For this review, take the finished solid that the model builds, in its own axes (mm). A direction names the side the tool comes from. Give positions to 0.01 mm unless a question says otherwise; leave off trailing zeros. Write each loop counter-clockwise with the first axis right and the second up, starting at its lowest first coordinate (ties: lowest second). Pieces come first, ordered by that corner, then holes. Notation, with made-up numbers: M 40.5,-22 L 64.5,-22 A28 ccw 64.5,-4 Z; hole C 9.25,-25.75 d2. An arc over 180 degrees is marked long. One line per item, written item: value. Start each with the question number.
Item 1: Clearance check with flat-ended pins moving along their axes: pin 1 Ø2 at (y, z) = (0.5, -5) entering from -X; pin 2 Ø8 at (x, z) = (6, 2) entering from +Y; pin 3 Ø2 at (x, y) = (5, 1.5) entering from +Z; pin 4 Ø2 at (x, y) = (2, 0.5) entering from +Z. State where each tip first meets the part, or that it passes through.
Item 2: Consider section B-B, the plane x = 0. Write out the cut boundary in (y, z), and give its area (3 significant figures).
Item 3: Consider section A-A, the plane z = 0. Write out the cut boundary in (x, y), and give its area (3 significant figures).
Item 4: To check wall thickness, follow probe 1 along Z at (x, y) = (0, 3.45); probe 2 along Z at (x, y) = (0, 1.2). State the ranges of each line that lie inside material, in increasing order.
Item 5: Tool access review of faces 4 (the face through (6, 3.4, -2)), 5 (the face through (6, 0.1, -2)), 6 (the face through (7, 3.5, -2)): name each direction out of +Z, -Z, +X, -X, +Y, -Y from which nothing blocks a thin tool from reaching the whole face with its end or side.
Item 6: Mouldability with a two-part tool opening along X and no side actions: class faces 1 (the face through (-4, 0, -4)), 2 (the face through (-7.493, 1.726, -0.33)), 3 (the face through (-1.08, 1.73, 4.88)) as released by +X, released by -X, zero draft, split by the parting line, or undercut.
Item 7: Consider section C-C, the plane y = 2. Write out the cut boundary in (x, z), and give its area (3 significant figures).
Item 8: Consider section D-D, the plane z = 6.75. Write out the cut boundary in (x, y), and give its area (3 significant figures).
```python
from build123d import *

# Parameters (mm, degrees)
SKETCH1_R           = 7.5
SKETCH1_R_2         = 7
BOSS_EXTRUDE1_DEPTH = 3.5
SKETCH6_R           = 7
SKETCH6_R_2         = 6
BOSS_EXTRUDE4_DEPTH = 3.3
SKETCH7_R           = 6
SKETCH7_R_2         = 5
BOSS_EXTRUDE5_DEPTH = 3.5


with BuildPart() as part:
    # Sketch1 → Boss-Extrude1 (new body)
    with BuildSketch(Plane(origin=(0, 0, 0), x_dir=(1, 0, 0), z_dir=(0, 1, 0))):
        Circle(SKETCH1_R)
        Circle(SKETCH1_R_2, mode=Mode.SUBTRACT)
    extrude(amount=BOSS_EXTRUDE1_DEPTH)

    # Sketch6 → Boss-Extrude4 (add)
    with BuildSketch(Plane(origin=(0, 0.1, 0), x_dir=(1, 0, 0), z_dir=(0, 1, 0))):
        Circle(SKETCH6_R)
        Circle(SKETCH6_R_2, mode=Mode.SUBTRACT)
    extrude(amount=BOSS_EXTRUDE4_DEPTH)

    # Sketch7 → Boss-Extrude5 (add)
    with BuildSketch(Plane(origin=(0, 0, 0), x_dir=(1, 0, 0), z_dir=(0, 1, 0))):
        Circle(SKETCH7_R)
        Circle(SKETCH7_R_2, mode=Mode.SUBTRACT)
    extrude(amount=BOSS_EXTRUDE5_DEPTH)


solid = part.part
```
Model answer:
1. pin 1: stops at x = -6.34
1. pin 2: stops at y = 3.5
1. pin 3: stops at z = 6.34
1. pin 4: stops at z = 7.43
2. outline: M 0,-7.5 L 3.5,-7.5 L 3.5,-7 L 3.4,-7 L 3.4,-6 L 3.5,-6 L 3.5,-5 L 0,-5 L 0,-6 L 0.1,-6 L 0.1,-7 L 0,-7 Z; M 0,5 L 3.5,5 L 3.5,6 L 3.4,6 L 3.4,7 L 3.5,7 L 3.5,7.5 L 0,7.5 L 0,7 L 0.1,7 L 0.1,6 L 0,6 Z
2. area: 17.1 mm2
3. outline: M -7.5,0 L -7,0 L -7,0.1 L -6,0.1 L -6,0 L -5,0 L -5,3.5 L -6,3.5 L -6,3.4 L -7,3.4 L -7,3.5 L -7.5,3.5 Z; M 5,0 L 6,0 L 6,0.1 L 7,0.1 L 7,0 L 7.5,0 L 7.5,3.5 L 7,3.5 L 7,3.4 L 6,3.4 L 6,3.5 L 5,3.5 Z
3. area: 17.1 mm2
4. probe 1: z = -7.5 to -7, -6 to -5, 5 to 6, 7 to 7.5
4. probe 2: z = -7.5 to -5, 5 to 7.5
5. face 4: +Y
5. face 5: -Y
5. face 6: +Z, -Z, +X, -X, +Y
6. face 1: zero draft
6. face 2: split by the parting line
6. face 3: undercut
7. outline: C 0,0 d15; hole C 0,0 d10
7. area: 98.2 mm2
8. outline: M -3.27,0 L -1.85,0 L -1.85,0.1 L 1.85,0.1 L 1.85,0 L 3.27,0 L 3.27,3.5 L 1.85,3.5 L 1.85,3.4 L -1.85,3.4 L -1.85,3.5 L -3.27,3.5 Z
8. area: 22.1 mm2
